Geometry check sheet. Reference: drawing and pictorial views, mm from the part's lowest x, y, z. Round coordinates to 2 decimals unless told otherwise and drop trailing zeros. Order: outer loops, then holes, each group sorted by start corner. A loop starts at its lowest first (then second) coordinate and runs counter-clockwise, first axis right, second up. Notation, with made-up numbers: (4, 62.25) -> (27, 62.25) arc R33 ccw to (27, 96.25) -> close; hole circle Ø7 at (79.25, 46.25). An arc over 180 degrees is marked (long way). Put each result on its own line as item: value.
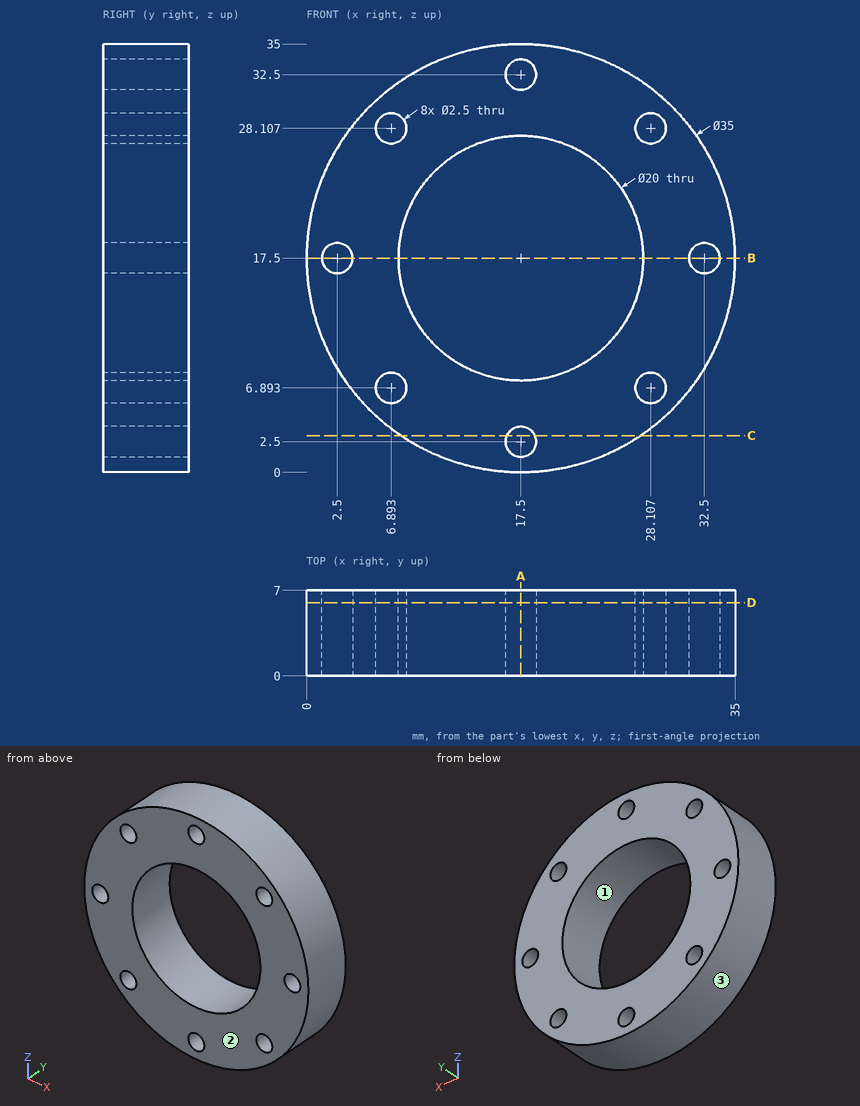
Item 1: Depth check by flat-ended pin: pin 1 Ø2 at (x, y) = (24.5, 3.5) entering from -Z; pin 2 Ø2 at (x, z) = (28.11, 28.11) entering from -Y; pin 3 Ø3 at (x, y) = (28.5, 2.5) entering from +Z; pin 4 Ø4 at (y, z) = (2, 8) entering from -X. Enter the tip coordinate at first touch or a pass-through.
Geometry check:
pin 1: z = 1.06
pin 2: through
pin 3: z = 32.2
pin 4: x = 1.69
Item 2: Sectioned sample at B-B, the plane z = 17.5. Record the boundary of the cut face in (x, y).
Geometry check:
outline: (0, 0) -> (1.25, 0) -> (1.25, 7) -> (0, 7) -> close; (3.75, 0) -> (7.5, 0) -> (7.5, 7) -> (3.75, 7) -> close; (27.5, 0) -> (31.25, 0) -> (31.25, 7) -> (27.5, 7) -> close; (33.75, 0) -> (35, 0) -> (35, 7) -> (33.75, 7) -> close
Item 3: Sectioned sample at A-A, the plane x = 17.5. Record the boundary of the cut face in (y, z).
Geometry check:
outline: (0, 0) -> (7, 0) -> (7, 1.25) -> (0, 1.25) -> close; (0, 3.75) -> (7, 3.75) -> (7, 7.5) -> (0, 7.5) -> close; (0, 27.5) -> (7, 27.5) -> (7, 31.25) -> (0, 31.25) -> close; (0, 33.75) -> (7, 33.75) -> (7, 35) -> (0, 35) -> close
Item 4: Material ranges on line 1 along Z through (x, y) = (17.5, 3.5); line 2 along Z through (x, y) = (6.5, 1.5) (1 decimal), recorded low to high.
Geometry check:
line 1: 0 to 1.25, 3.75 to 7.5, 27.5 to 31.25, 33.75 to 35
line 2: 3.9 to 5.7, 8.1 to 26.9, 29.3 to 31.1
Item 5: Release check for a two-part mould opening along Z. For the marked faces 1, 2 and 3 record: pulls with the +Z half, pulls with the -Z half, needs draft (parallel to the pull), parting line crosses it, or undercut.
Geometry check:
face 1: undercut
face 2: needs draft
face 3: parting line crosses it
Item 6: Sectioned sample at C-C, the plane z = 3. Record the boundary of the cut face in (x, y) (1 decimal).
Geometry check:
outline: (7.7, 0) -> (16.4, 0) -> (16.4, 7) -> (7.7, 7) -> close; (18.6, 0) -> (27.3, 0) -> (27.3, 7) -> (18.6, 7) -> close
Item 7: Sectioned sample at D-D, the plane y = 6. Give the number of separate pieces and of enclosed holes in the cut face.
Geometry check:
separate pieces: 1
enclosed holes: 9
